from build123d import *

# Parameters (mm, degrees)
CYLINDER023_R               = 3.6
CYLINDER023_DEPTH           = 8
CYLINDER023_ROLL_ANGLE      = 89.941329
CYLINDER023_PITCH_ANGLE     = 3.606623
CYLINDER023_PLACEMENT_ANGLE = -0.059115
PAD031_DEPTH                = 3
SKETCH032_W                 = 40.456886
SKETCH032_H                 = 21.390591
PAD032_DEPTH                = 5
CYLINDER024_R               = 1.1
CYLINDER024_DEPTH           = 10
CYLINDER025_R               = 1.1
CYLINDER025_DEPTH           = 10
SKETCH035_W                 = 23.3
SKETCH035_H                 = 12.5
PAD035_DEPTH                = 19.5
SKETCH033_W                 = 32.5
SKETCH033_H                 = 12.5
PAD034_DEPTH                = 4.5
SKETCH034_W                 = 36.061928
SKETCH034_H                 = 25.639376
PAD033_DEPTH                = 14
CUT030_PLACEMENT_ANGLE      = 90


with BuildPart() as cylinder023:
    # Cylinder023 → Cylinder023 (new body)
    with BuildSketch(Plane.XY):
        Circle(CYLINDER023_R)
    extrude(amount=CYLINDER023_DEPTH)


with BuildPart() as cylinder023_1:
    # Cylinder023 roll: moved
    add(cylinder023.part.rotate(Axis((0, 0, 0), (1, 0, 0)), CYLINDER023_ROLL_ANGLE))


with BuildPart() as cylinder023_2:
    # Cylinder023 pitch: moved
    add(cylinder023_1.part.rotate(Axis((0, 0, 0), (0, 1, 0)), CYLINDER023_PITCH_ANGLE))


with BuildPart() as cylinder023_3:
    # Cylinder023 placement: moved
    add(cylinder023_2.part.moved(Location((21, 34, 6.3))).rotate(Axis((21, 34, 6.3), (0, 0, 1)), CYLINDER023_PLACEMENT_ANGLE))


with BuildPart() as obj1:
    # Sketch031 → Pad031 (new body)
    with BuildSketch(Plane.XZ):
        with BuildLine():
            ThreePointArc((-18.00002, 2), (-20, 0), (-18.00002, -2))
            Line((-18.00002, -2), (-2.073587, -3.25))
            ThreePointArc((-2.073587, -3.25), (0, -3.854383), (2.073587, -3.25))
            Line((2.073587, -3.25), (18.00002, -2))
            ThreePointArc((18.00002, -2), (20, 0), (18.00002, 2))
            Line((2.073587, 3.25), (18.00002, 2))
            ThreePointArc((2.073587, 3.25), (0, 3.862152), (-2.073587, 3.25))
            Line((-18.00002, 2), (-2.073587, 3.25))
        make_face()
    extrude(amount=PAD031_DEPTH)


with BuildPart() as obj1_1:
    # Body034 placement: moved
    add(obj1.part.moved(Location((21, 35, 6.3))))

    # Fusion026: union Cylinder023
    add(cylinder023_3.part)


with BuildPart() as obj1_2:
    # Fusion026 placement: moved
    add(obj1_1.part.moved(Location((-21, -35, 4))))


with BuildPart() as cut027:
    # Sketch032 → Pad032 (new body)
    with BuildSketch(Plane.XZ):
        with Locations((0, 10.695296)):
            Rectangle(SKETCH032_W, SKETCH032_H)
    extrude(amount=PAD032_DEPTH)

    # Cut027: cut obj1
    add(obj1_2.part, mode=Mode.SUBTRACT)


with BuildPart() as cylinder024:
    # Cylinder024 → Cylinder024 (new body)
    with BuildSketch(Plane(origin=(30, 22, 6), x_dir=(1, 0, 0), z_dir=(0, -1, 0))):
        Circle(CYLINDER024_R)
    extrude(amount=CYLINDER024_DEPTH)


with BuildPart() as obj2:
    # Cylinder025 → Cylinder025 (new body)
    with BuildSketch(Plane(origin=(2.2, 22, 6), x_dir=(1, 0, 0), z_dir=(0, -1, 0))):
        Circle(CYLINDER025_R)
    extrude(amount=CYLINDER025_DEPTH)

    # Fusion027: union Cylinder024
    add(cylinder024.part)


with BuildPart() as cortecuerpo005:
    # Sketch035 → Pad035 (new body)
    with BuildSketch(Plane.XZ):
        with Locations((16.4, 6.25)):
            Rectangle(SKETCH035_W, SKETCH035_H)
    extrude(amount=PAD035_DEPTH)


with BuildPart() as cortecuerpo005_1:
    # Body038 placement: moved
    add(cortecuerpo005.part.moved(Location((0, 19, 0))))


with BuildPart() as cortetornillos005:
    # Sketch033 → Pad034 (new body)
    with BuildSketch(Plane.XZ):
        with Locations((16.25, 6.25)):
            Rectangle(SKETCH033_W, SKETCH033_H)
    extrude(amount=PAD034_DEPTH)


with BuildPart() as cortetornillos005_1:
    # Body037 placement: moved
    add(cortetornillos005.part.moved(Location((0, 23, 0))))


with BuildPart() as fusion028:
    # Sketch034 → Pad033 (new body)
    with BuildSketch(Plane.XY):
        with Locations((15.881367, 9.413649)):
            Rectangle(SKETCH034_W, SKETCH034_H)
    extrude(amount=PAD033_DEPTH)


with BuildPart() as fusion028_1:
    # Body036 placement: moved
    add(fusion028.part.moved(Location((0, 0, -1))))

    # Cut028: cut CorteTornillos005
    add(cortetornillos005_1.part, mode=Mode.SUBTRACT)

    # Cut029: cut CorteCuerpo005
    add(cortecuerpo005_1.part, mode=Mode.SUBTRACT)

    # Cut030: cut obj2
    add(obj2.part, mode=Mode.SUBTRACT)


with BuildPart() as fusion028_2:
    # Cut030 placement: moved
    add(fusion028_1.part.moved(Location((-15.5, -9.5, -2.5))).rotate(Axis((-15.5, -9.5, -2.5), (-1, 0, 0)), CUT030_PLACEMENT_ANGLE))

    # Fusion028: union Cut027
    add(cut027.part)


solid = fusion028_2.part
Can you work these out from the model? Positions are in its coordinate system, mm. A direction names the side the tool comes from. Round coordinates to 2 decimals unless told otherwise and drop trailing zeros. Write each loop counter-clockwise with the first axis right and the second up, starting at its lowest first coordinate (ties: lowest second). Pieces come first, ordered by that corner, then holes. Notation, with made-up numbers: (-19.5, 23.5) -> (-15.5, 23.5) arc R9 ccw to (-15.5, 39.5) -> close; hole circle Ø6 at (-33.5, 20.5). An arc over 180 degrees is marked (long way). Use one line per item in the form item = value. Start each with the question number.
Q1. I'm going to push flat-ended pins straight in: P1, Ø4, axis at x = -5, y = -5.5, coming from the -Z side; P2, Ø4, axis at y = -5, z = -23.5, coming from the -X side; P3, Ø1, axis at x = 1.5, z = 3, coming from the -Y side. Where does each tip first touch, or does it pass through?
Q2. Imagine slicing it at A-A (y = -6.25). Please give me the cut outline in (x, z), then the cut area to 3 significant figures.
Q3. Imagine slicing it at C-C (z = 4). Please give me the cut outline in (x, y), then the cut area to 3 significant figures.
Q4. Which directions (+Z, -Z, +X, -X, +Y, -Y) give clear straight access to the entire face, cutting with the end or side of a thin tool? Please do faces 4 (the face through (19, -2, 0)), 5 (the face through (20, -1.5, 10.3)), 6 (the face through (-10.75, -3, -12)), 7 (the face through (-19, -2, 0)).
Q5. Imagine slicing it at D-D (x = 14.5). Please give me the cut outline in (y, z).
Q6. If I drill on probe 1 along X at (y, z) = (-3.5, -15.75); probe 2 along X at (y, z) = (-6.25, -2.5); probe 3 along X at (y, z) = (-4, -22), over which ranges is the centre line in solid material (lowest first)? Write a range as [from, to].
Q7. We'd pull the mould along X, two halves only. Please class faces 1 (the face through (20.228, -2, 11)), 2 (the face through (0, 2, 0.906)), 3 (the face through (2.12, -3.98, 13.21)): +X half, -X half, draft (parallel to the pull), parting line (faces both ways), or undercut.
Q8. Imagine slicing it at B-B (x = -11.5). Please give me the cut outline in (y, z), then the cut area to 3 significant figures.
Worked out:
q1.P1 = -2
q1.P2 = -17.65
q1.P3 = -5
q2.outline = (-17.65, -24.73) -> (-15.5, -24.73) -> (-15.5, -21) -> (-10.75, -21) -> (-10.75, -2) -> (12.55, -2) -> (12.55, -21) -> (17, -21) -> (17, -24.73) -> (18.41, -24.73) -> (18.41, 0.91) -> (-17.65, 0.91) -> close
q2.area = 361 mm^2
q3.outline = (-20.23, -5) -> (20.23, -5) -> (20.23, 0) -> (-20.23, 0) -> close
q3.area = 202 mm^2
q4.face_4 = -Z, +X, +Y, -Y
q4.face_5 = +Y
q4.face_6 = -Z
q4.face_7 = -Z, -X, +Y, -Y
q5.outline = (-10.5, -24.73) -> (-9.5, -24.73) -> (-9.5, -21) -> (-4.6, -21) -> (-4.6, -14.5) -> (-2.4, -14.5) -> (-2.4, -21) -> (3, -21) -> (3, -24.73) -> (3.5, -24.73) -> (3.5, 0.91) -> (0, 0.91) -> (0, 8.03) -> (-3, 8.03) -> (-3, 12.57) -> (0, 12.57) -> (0, 21.39) -> (-5, 21.39) -> (-5, 0.91) -> (-10.5, 0.91) -> close
q6.probe_1 = [-17.65, -14.4], [-12.2, -10.75], [12.55, 13.4], [15.6, 18.41]
q6.probe_2 = [-17.65, -10.75], [12.55, 18.41]
q6.probe_3 = [-17.65, -15.5], [17, 18.41]
q7.face_1 = +X half
q7.face_2 = draft
q7.face_3 = undercut
q8.outline = (-10.5, -24.73) -> (-9.5, -24.73) -> (-9.5, -21) -> (3, -21) -> (3, -24.73) -> (3.5, -24.73) -> (3.5, 0.91) -> (0, 0.91) -> (0, 7.79) -> (-3, 7.79) -> (-3, 12.81) -> (0, 12.81) -> (0, 21.39) -> (-5, 21.39) -> (-5, 0.91) -> (-10.5, 0.91) -> close
q8.area = 400 mm^2
